from build123d import *

# Parameters (mm, degrees)
SKETCH1_W           = 14
SKETCH1_H           = 8
BOSS_EXTRUDE1_DEPTH = 1
SKETCH2_W           = 12
SKETCH2_H           = 7
BOSS_EXTRUDE2_DEPTH = 4
FILLET2_R           = 3.3
FILLET1_R           = 3.5


with BuildPart() as part:
    # Sketch1 → Boss-Extrude1 (new body)
    with BuildSketch(Plane.XY):
        Rectangle(SKETCH1_W, SKETCH1_H)
    extrude(amount=BOSS_EXTRUDE1_DEPTH)

    # Sketch2 → Boss-Extrude2 (add)
    with BuildSketch(Plane.XY.offset(1)):
        Rectangle(SKETCH2_W, SKETCH2_H)
    extrude(amount=BOSS_EXTRUDE2_DEPTH)

    # Fillet2
    fillet2_edges = [part.edges().sort_by_distance(p)[0] for p in [
        (6, -3.5, 3),
        (6, 3.5, 3),
        (-6, 3.5, 3),
        (-6, -3.5, 3),
    ]]
    fillet(fillet2_edges, radius=FILLET2_R)

    # Fillet1
    fillet1_edges = [part.edges().sort_by_distance(p)[0] for p in [
        (7, -4, 0.5),
        (-7, -4, 0.5),
        (-7, 4, 0.5),
        (7, 4, 0.5),
    ]]
    fillet(fillet1_edges, radius=FILLET1_R)


solid = part.part
Model file for the job. Use its own axes, mm. A direction names the side the tool comes from. Give positions to 0.01 mm unless a question says otherwise; leave off trailing zeros. Loops run counter-clockwise (first coordinate to the right, second up) from the corner with the lowest first, then second, coordinate; pieces in that order, holes last.
Item 1: Which spindle directions (+Z, -Z, +X, -X, +Y, -Y) get a long thin tool onto all of the face, cutting with end or side? Do faces 1 (the face through (0, -3.5, 3)), 2 (the face through (5.008, -2.559, 3.028)), 3 (the face through (-5.008, 2.559, 3.028)), 4 (the face through (0, 3.5, 3)). Say none if no direction does.
Check values:
face 1: +Z, +X, -X, -Y
face 2: +Z, +X, -Y
face 3: +Z, -X, +Y
face 4: +Z, +X, -X, +Y
Item 2: Slice it at A-A (z = 3.1). Write the cut outline in (x, y).
Check values:
outline: (-6, -0.2) arc R3.3 ccw to (-2.7, -3.5) - (2.7, -3.5) arc R3.3 ccw to (6, -0.2) - (6, 0.2) arc R3.3 ccw to (2.7, 3.5) - (-2.7, 3.5) arc R3.3 ccw to (-6, 0.2) - close
Item 3: Drop a flat-ended pin along its axis: P1, Ø1.2, axis at x = 0.5, z = 3.5, coming from the +Y side. Give the stop position or say it passes through.
Check values:
P1: stops at y = 3.5
Item 4: Slice it at B-B (x = -0.75). Write the cut outline in (y, z), plus the area to 3 significant figures.
Check values:
outline: (-4, 0) - (4, 0) - (4, 1) - (3.5, 1) - (3.5, 5) - (-3.5, 5) - (-3.5, 1) - (-4, 1) - close
area: 36.0 mm2
Item 5: Drill centre lines: line 1 along Y through (x, z) = (1, 1.55); line 2 along Z through (x, y) = (-6, 1.25); line 3 along Y through (x, z) = (-4.25, 4.7). Where is each one in solid material? Low to high.
Check values:
line 1: y = -3.5 to 3.5
line 2: z = 0 to 1
line 3: y = -3.11 to 3.11
